Part model, mm, in its own coordinate system. A direction names the side the tool comes from. Give positions to 0.01 mm unless a question says otherwise; leave off trailing zeros. Write each loop counter-clockwise with the first axis right and the second up, starting at its lowest first coordinate (ties: lowest second). Pieces come first, ordered by that corner, then holes. Notation, with made-up numbers: M 50,-24 L 72,-24 A25 cw 72,8 Z; hole C 45,52 d4. An arc over 180 degrees is marked long. Use a Markdown table: item, result. Add a question column.
from build123d import *

# Parameters (mm, degrees)
IZIM1_W                     = 140
IZIM1_H                     = 140
IZIM1_R                     = 9
Y_KSEKLIK_EKSTR_ZYON1_DEPTH = 20
KES_EKSTR_ZYON1_DEPTH       = 10
KES_EKSTR_ZYON2_DEPTH       = 101.995049384


with BuildPart() as part:
    # Çizim1 → Yükseklik-Ekstrüzyon1 (new body)
    with BuildSketch(Plane(origin=(0, 0, 0), x_dir=(1, 0, 0), z_dir=(0, 1, 0))):
        Rectangle(IZIM1_W, IZIM1_H)
        with Locations(Location((-50, 50, 0), (0, 0, 270))):
            Circle(IZIM1_R, mode=Mode.SUBTRACT)
        with Locations(Location((50, 50, 0), (0, 0, 270))):
            Circle(IZIM1_R, mode=Mode.SUBTRACT)
        with Locations(Location((-50, -50, 0), (0, 0, 270))):
            Circle(IZIM1_R, mode=Mode.SUBTRACT)
        with Locations(Location((50, -50, 0), (0, 0, 270))):
            Circle(IZIM1_R, mode=Mode.SUBTRACT)
    extrude(amount=-Y_KSEKLIK_EKSTR_ZYON1_DEPTH)

    # Çizim4 → Kes-Ekstrüzyon1 (cut)
    # profile 1 of 2: a face of its own
    with BuildSketch(Plane(origin=(0, 0, 0), x_dir=(1, 0, 0), z_dir=(0, 1, 0))):
        with BuildLine():
            Line((-5, 20.227170593), (-5, -19.772829407))
            ThreePointArc((-5, -19.772829407), (-20, -34.772829407), (-35, -19.772829407))
            Line((-35, -19.772829407), (-35, 20.227170593))
            ThreePointArc((-35, 20.227170593), (-20, 35.227170593), (-5, 20.227170593))
        make_face()
        with BuildLine():
            Line((-30, 20.227170593), (-30, -19.772829407))
            ThreePointArc((-30, -19.772829407), (-20, -29.772829407), (-10, -19.772829407))
            Line((-10, -19.772829407), (-10, 20.227170593))
            ThreePointArc((-10, 20.227170593), (-20, 30.227170593), (-30, 20.227170593))
        make_face(mode=Mode.SUBTRACT)
    # profile 2 of 2: a face of its own
    with BuildSketch(Plane(origin=(0, 0, 0), x_dir=(1, 0, 0), z_dir=(0, 1, 0))):
        with BuildLine():
            Line((35, 20), (35, -20))
            ThreePointArc((35, -20), (20, -35), (5, -20))
            Line((5, -20), (5, 20))
            ThreePointArc((5, 20), (20, 35), (35, 20))
        make_face()
        with BuildLine():
            Line((30, 20), (30, -20))
            ThreePointArc((30, -20), (20, -30), (10, -20))
            Line((10, -20), (10, 20))
            ThreePointArc((10, 20), (20, 30), (30, 20))
        make_face(mode=Mode.SUBTRACT)
    extrude(amount=-KES_EKSTR_ZYON1_DEPTH, mode=Mode.SUBTRACT)

    # Çizim2 → Kes-Ekstrüzyon2 (cut, through all)
    with BuildSketch(Plane(origin=(0, -20, 0), x_dir=(-1, 0, 0), z_dir=(0, -1, 0))):
        with BuildLine():
            Line((-10, 20), (-10, -20))
            ThreePointArc((-10, -20), (-20, -30), (-30, -20))
            Line((-30, -20), (-30, 20))
            ThreePointArc((-30, 20), (-20, 30), (-10, 20))
        make_face()
        with BuildLine():
            Line((30, 20.227170593), (30, -19.772829407))
            ThreePointArc((30, -19.772829407), (20, -29.772829407), (10, -19.772829407))
            Line((10, -19.772829407), (10, 20.227170593))
            ThreePointArc((10, 20.227170593), (20, 30.227170593), (30, 20.227170593))
        make_face()
    extrude(amount=-KES_EKSTR_ZYON2_DEPTH, mode=Mode.SUBTRACT)

    # Çizim6 → #6-40 Dişli Delik1 (revolve, cut)
    with BuildSketch(Plane(origin=(0, 0, -40.730803154), x_dir=(0, 0, 1), z_dir=(1, 0, 0))):
        Polygon((0, 0), (0, 20), (2.3876, 20), (1.4351, 19.0475), (1.4351, 0), align=None)
    revolve(axis=Axis((0, 6.35, -40.730803154), (0, -1, 0)), mode=Mode.SUBTRACT)


solid = part.part
1. Flat gauge pins, fed straight in: pin 1 (16 mm diameter, centred on x = -50, z = 50, fed in from -Y); pin 2 (15 mm diameter, centred on x = -15, z = 3.5, fed in from +Y). Where does each tip first touch, or does it go through?
2. Cut at C-C (y = -2). Write the cut outline in (x, z), then the cut area to 3 significant figures.
3. Cut at B-B (x = -50). Write the cut outline in (y, z).
4. Drill centre lines: probe 1 along X at (y, z) = (-9, 18.5); probe 2 along X at (y, z) = (-11, 50); probe 3 along Z at (x, y) = (0, -6.5). Where is each one in solid material? Low to high. Write a range as [from, to].
5. Mould opens along Z. For faces 4 (the flat face through (-1, -20, -1)), 5 (the cylindrical face through (20, -15, 30)), 6 (the flat face through (-1, -10, -70)) say: released by +Z, released by -Z, zero draft, split by the parting line, or undercut.
6. Tool access for faces 1 (the flat face through (-30, -15, -1)), 2 (the cylindrical face through (-19.67, -4.93, 34.77)), 3 (the flat face through (-1, 0, -1)): list every direction of +Z, -Z, +X, -X, +Y, -Y with a clear straight run to the whole face (end or side of a thin tool).
7. Cut at A-A (z = -10.5). Write the cut outline in (x, y).
8. Cut at D-D (z = -50). Write the cut outline in (x, y), then the cut area to 3 significant figures.
A:
| question | item | result |
|---|---|---|
| 1 | pin 1 | passes through |
| 1 | pin 2 | stops at y = -10 |
| 2 | outline | M -70,-70 L 70,-70 L 70,70 L -70,70 Z; hole C -50,-50 d18; hole C -50,50 d18; hole M -35,-20.23 A15 ccw -5,-20.23 L -5,19.77 A15 ccw -35,19.77 Z; hole C 0,-40.73 d2.87; hole M 5,-20 A15 ccw 35,-20 L 35,20 A15 ccw 5,20 Z; hole C 50,-50 d18; hole C 50,50 d18 |
| 2 | area | 14,800 mm² |
| 3 | outline | M -20,-70 L 0,-70 L 0,-59 L -20,-59 Z; M -20,-41 L 0,-41 L 0,41 L -20,41 Z; M -20,59 L 0,59 L 0,70 L -20,70 Z |
| 4 | probe 1 | x = [-70, -35], [-5, 5], [35, 70] |
| 4 | probe 2 | x = [-70, -59], [-41, 41], [59, 70] |
| 4 | probe 3 | z = [-70, -42.17], [-39.3, 70] |
| 5 | face 4 | zero draft |
| 5 | face 5 | undercut |
| 5 | face 6 | released by -Z |
| 6 | face 1 | +Y, -Y |
| 6 | face 2 | +Y |
| 6 | face 3 | +Z, -Z, +X, -X, +Y |
| 7 | outline | M -70,-20 L -30,-20 L -30,-10 L -35,-10 L -35,0 L -70,0 Z; M -10,-20 L 10,-20 L 10,-10 L 5,-10 L 5,0 L -5,0 L -5,-10 L -10,-10 Z; M 30,-20 L 70,-20 L 70,0 L 35,0 L 35,-10 L 30,-10 Z |
| 8 | outline | M -70,-20 L -59,-20 L -59,0 L -70,0 Z; M -41,-20 L 41,-20 L 41,0 L -41,0 Z; M 59,-20 L 70,-20 L 70,0 L 59,0 Z |
| 8 | area | 2,080 mm² |
